```python
from build123d import *

# Parameters (mm, degrees)
F0_W     = 1820
F0_H     = 1820
F1_DEPTH = 390
F2_W     = 330
F2_H     = 330
F2_H_2   = 157.5
F2_W_2   = 15
F3_DEPTH = 740.61349
F4_DEPTH = 5


with BuildPart() as f1:
    # F0 (on Front) → F1 (new body)
    with BuildSketch(Plane.XZ):
        with Locations((910, 910)):
            Rectangle(F0_W, F0_H)
    extrude(amount=F1_DEPTH)

    # F2 (on Front) → F3 (cut)
    with BuildSketch(Plane.XZ):
        with Locations((220, 220)):
            Rectangle(F2_W, F2_H)
        with Locations((220, 565)):
            Rectangle(F2_W, F2_H)
        with Locations((220, 910)):
            Rectangle(F2_W, F2_H)
        with Locations((220, 1255)):
            Rectangle(F2_W, F2_H)
        with Locations((220, 1600)):
            Rectangle(F2_W, F2_H)
        with Locations((565, 220)):
            Rectangle(F2_W, F2_H)
        with Locations((565, 1600)):
            Rectangle(F2_W, F2_H)
        with Locations((910, 220)):
            Rectangle(F2_W, F2_H)
        with Locations((910, 1600)):
            Rectangle(F2_W, F2_H)
        with Locations((1255, 220)):
            Rectangle(F2_W, F2_H)
        with Locations((1255, 1600)):
            Rectangle(F2_W, F2_H)
        with Locations((1600, 220)):
            Rectangle(F2_W, F2_H)
        with Locations((1600, 565)):
            Rectangle(F2_W, F2_H)
        with Locations((1600, 910)):
            Rectangle(F2_W, F2_H)
        with Locations((1600, 1255)):
            Rectangle(F2_W, F2_H)
        with Locations((1600, 1600)):
            Rectangle(F2_W, F2_H)
        with Locations((565, 910)):
            Rectangle(F2_W, F2_H)
        with Locations((565, 1255)):
            Rectangle(F2_W, F2_H)
        with Locations((910, 910)):
            Rectangle(F2_W, F2_H)
        with Locations((910, 1255)):
            Rectangle(F2_W, F2_H)
        with Locations((1255, 910)):
            Rectangle(F2_W, F2_H)
        with Locations((1255, 1255)):
            Rectangle(F2_W, F2_H)
        with Locations((565, 651.25)):
            Rectangle(F2_W, F2_H_2)
        with Locations((565, 478.75)):
            Rectangle(F2_W, F2_H_2)
        with Locations((1255, 651.25)):
            Rectangle(F2_W, F2_H_2)
        with Locations((1255, 478.75)):
            Rectangle(F2_W, F2_H_2)
        with Locations((737.5, 651.25)):
            Rectangle(F2_W_2, F2_H_2)
        with Locations((737.5, 478.75)):
            Rectangle(F2_W_2, F2_H_2)
        with Locations((910, 651.25)):
            Rectangle(F2_W, F2_H_2)
        with Locations((1082.5, 651.25)):
            Rectangle(F2_W_2, F2_H_2)
        with Locations((910, 478.75)):
            Rectangle(F2_W, F2_H_2)
        with Locations((1082.5, 478.75)):
            Rectangle(F2_W_2, F2_H_2)
        Polygon((400, 1075), (730, 1075), (730, 745), (745, 745), (745, 1075), (1075, 1075), (1075, 745), (1090, 745), (1090, 1075), (1420, 1075), (1420, 1090), (1090, 1090), (1090, 1420), (1075, 1420), (1075, 1090), (745, 1090), (745, 1420), (730, 1420), (730, 1090), (400, 1090), align=None)
    extrude(amount=F3_DEPTH, mode=Mode.SUBTRACT)

    # F2 (on Front) → F4 (join)
    with BuildSketch(Plane.XZ):
        with Locations((565, 478.75)):
            Rectangle(F2_W, F2_H_2)
        with Locations((565, 651.25)):
            Rectangle(F2_W, F2_H_2)
        with Locations((910, 651.25)):
            Rectangle(F2_W, F2_H_2)
        with Locations((910, 478.75)):
            Rectangle(F2_W, F2_H_2)
        with Locations((1255, 478.75)):
            Rectangle(F2_W, F2_H_2)
        with Locations((1255, 651.25)):
            Rectangle(F2_W, F2_H_2)
        with Locations((565, 910)):
            Rectangle(F2_W, F2_H)
        with Locations((1255, 910)):
            Rectangle(F2_W, F2_H)
        with Locations((1255, 1255)):
            Rectangle(F2_W, F2_H)
        with Locations((910, 1255)):
            Rectangle(F2_W, F2_H)
        with Locations((565, 1255)):
            Rectangle(F2_W, F2_H)
        with Locations((910, 910)):
            Rectangle(F2_W, F2_H)
        Polygon((400, 1075), (730, 1075), (730, 745), (745, 745), (745, 1075), (1075, 1075), (1075, 745), (1090, 745), (1090, 1075), (1420, 1075), (1420, 1090), (1090, 1090), (1090, 1420), (1075, 1420), (1075, 1090), (745, 1090), (745, 1420), (730, 1420), (730, 1090), (400, 1090), align=None)
        with Locations((737.5, 651.25)):
            Rectangle(F2_W_2, F2_H_2)
        with Locations((737.5, 478.75)):
            Rectangle(F2_W_2, F2_H_2)
        with Locations((1082.5, 478.75)):
            Rectangle(F2_W_2, F2_H_2)
        with Locations((1082.5, 651.25)):
            Rectangle(F2_W_2, F2_H_2)
    extrude(amount=F4_DEPTH)


solid = f1.part
```
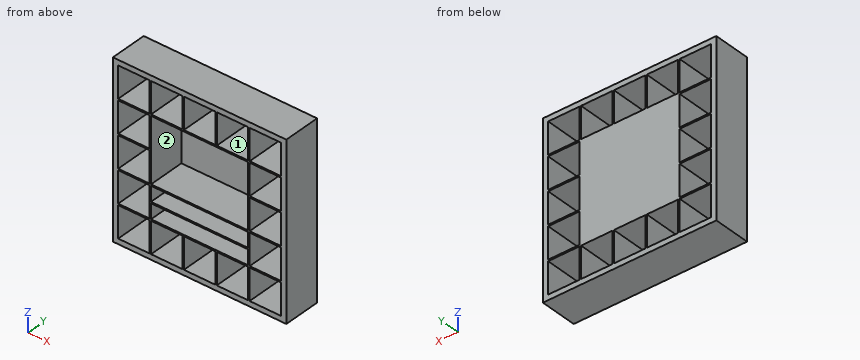
Design review of the part built by this model. Coordinates are the model's own, in mm. Face numbers are marked on the shaded views. A direction names the side the tool comes from. Coordinates: 2 decimals unless noted, no trailing zeros. Write each loop counter-clockwise with the first axis right and the second up, starting at its lowest first coordinate (ties: lowest second). Pieces come first, ordered by that corner, then holes.
1) Add section D-D (x = 1332). Write out the cut boundary in (y, z).
2) Add section B-B (z = 1680). Write out the cut boundary in (x, y).
3) To check wall thickness, follow L1, parallel to X at y = -373.5, z = 748.5; L2, parallel to Z at x = 773, y = -362; L3, parallel to X at y = -358.5, z = 301. State the ranges of each line that lie inside material, in increasing order.
4) Machinability: for the marked faces 1 and 2, which of the approach directions +Z, -Z, +X, -X, +Y, -Y give a long, thin tool a straight path to every point of the face, cutting with its end or side? Answer none if there is none.
5) Add section A-A (x = 131.5). Write out the cut boundary in (y, z).
6) Add section C-C (z = 443). Write out the cut boundary in (x, y).
Check result:
1. outline: (-390, 0) - (0, 0) - (0, 55) - (-390, 55) - close; (-390, 385) - (0, 385) - (0, 1435) - (-390, 1435) - (-390, 1420) - (-5, 1420) - (-5, 745) - (-390, 745) - (-390, 730) - (-5, 730) - (-5, 572.5) - (-390, 572.5) - (-390, 557.5) - (-5, 557.5) - (-5, 400) - (-390, 400) - close; (-390, 1765) - (0, 1765) - (0, 1820) - (-390, 1820) - close
2. outline: (0, -390) - (55, -390) - (55, 0) - (0, 0) - close; (385, -390) - (400, -390) - (400, 0) - (385, 0) - close; (730, -390) - (745, -390) - (745, 0) - (730, 0) - close; (1075, -390) - (1090, -390) - (1090, 0) - (1075, 0) - close; (1420, -390) - (1435, -390) - (1435, 0) - (1420, 0) - close; (1765, -390) - (1820, -390) - (1820, 0) - (1765, 0) - close
3. L1: x = 0 to 55, 385 to 400, 1420 to 1435, 1765 to 1820
3. L2: z = 0 to 55, 385 to 400, 557.5 to 572.5, 730 to 745, 1420 to 1435, 1765 to 1820
3. L3: x = 0 to 55, 385 to 400, 730 to 745, 1075 to 1090, 1420 to 1435, 1765 to 1820
4. face 1: +Y, -Y
4. face 2: -Y
5. outline: (-390, 0) - (0, 0) - (0, 55) - (-390, 55) - close; (-390, 385) - (0, 385) - (0, 400) - (-390, 400) - close; (-390, 730) - (0, 730) - (0, 745) - (-390, 745) - close; (-390, 1075) - (0, 1075) - (0, 1090) - (-390, 1090) - close; (-390, 1420) - (0, 1420) - (0, 1435) - (-390, 1435) - close; (-390, 1765) - (0, 1765) - (0, 1820) - (-390, 1820) - close
6. outline: (0, -390) - (55, -390) - (55, 0) - (0, 0) - close; (385, -390) - (400, -390) - (400, -5) - (1420, -5) - (1420, -390) - (1435, -390) - (1435, 0) - (385, 0) - close; (1765, -390) - (1820, -390) - (1820, 0) - (1765, 0) - close
